Here's how the part is built. I have some questions about the finished solid (model axes, mm). A direction names the side the tool comes from. Round coordinates to 2 decimals unless told otherwise and drop trailing zeros. Write each loop counter-clockwise with the first axis right and the second up, starting at its lowest first coordinate (ties: lowest second). Pieces come first, ordered by that corner, then holes. Notation, with made-up numbers: (22, 22.25) - (50, 22.25) arc R26 ccw to (50, 59.25) - close; hole circle Ø4 at (26, 37.25). An arc over 180 degrees is marked (long way). Use one line per item in the form item = value. Start each with the question number.
1. I want a section at B-B, the plane z = 2. List the corners of the cut face in (x, y) for me, plus the area to 3 significant figures.
2. Will these pins go through, and if not, where does the flat tip stop? pin 1 (1 mm diameter, centred on y = 3, z = 6, fed in from -X); pin 2 (5 mm diameter, centred on x = -5.5, z = 6.5, fed in from +Y).
3. If I drill on line 1 along X through (y, z) = (0.4, -1.5); line 2 along Y through (x, z) = (6.25, 4); line 3 along Z through (x, y) = (-9.5, 3.7), over which ranges is the centre line in solid material (lowest first)?
4. Which directions (+Z, -Z, +X, -X, +Y, -Y) give clear straight access to the entire face, cutting with the end or side of a thin tool? Please do faces 1 (the flat face through (0, 2, -8.65)), 2 (the flat face through (-12, 1.6, 0)), 3 (the flat face through (0, 0, 0)), 4 (the flat face through (-11, 4, -3.8)), 5 (the flat face through (-11, 4, 3.8)).
5. I want a section at A-A, the plane x = -8.25. List the corners of the cut face in (y, z) for me, plus the area to 3 significant figures.
6. I want a section at C-C, the plane y = 3.95. List the corners of the cut face in (x, z) for me.
7. I want a section at D-D, the plane z = -7.25. List the corners of the cut face in (x, y) for me, plus the area to 3 significant figures.
```python
from build123d import *

# Parameters (mm, degrees)
SKETCH_1_W      = 23
SKETCH_1_H      = 17.3
EXTRUDE_1_DEPTH = 3.5
SKETCH_2_W      = 5.700101794
SKETCH_2_H      = 7.6
EXTRUDE_2_DEPTH = 0.7
SKETCH_3_W      = 1.500050897
SKETCH_3_H      = 7.6
EXTRUDE_3_DEPTH = 1.9


with BuildPart() as part:
    # Эскиз1 → Бобышка-Вытянуть1 (new body)
    with BuildSketch(Plane(origin=(0, 0, 0), x_dir=(1, 0, 0), z_dir=(0, 1, 0))):
        Rectangle(SKETCH_1_W, SKETCH_1_H)
    extrude(amount=EXTRUDE_1_DEPTH)

    # Эскиз2 → Бобышка-Вытянуть2 (add)
    with BuildSketch(Plane(origin=(0, 3.5, 0), x_dir=(1, 0, 0), z_dir=(0, 1, 0))):
        with Locations((-10.15, 0)):
            Rectangle(SKETCH_2_W, SKETCH_2_H)
    extrude(amount=EXTRUDE_2_DEPTH)

    # Эскиз3 → Бобышка-Вытянуть3 (add)
    with BuildSketch(Plane.XZ.offset(-3.5)):
        with Locations((-12.250025449, 0)):
            Rectangle(SKETCH_3_W, SKETCH_3_H)
    extrude(amount=EXTRUDE_3_DEPTH)


solid = part.part
```
Model answer:
q1.outline = (-13, 1.6) - (-11.5, 1.6) - (-11.5, 0) - (11.5, 0) - (11.5, 3.5) - (-7.3, 3.5) - (-7.3, 4.2) - (-13, 4.2) - close
q1.area = 87.3 mm2
q2.pin_1 = -11.5
q2.pin_2 = 3.5
q3.line_1 = -11.5 to 11.5
q3.line_2 = 0 to 3.5
q3.line_3 = -3.8 to 3.8
q4.face_1 = -Z, +X, -X, +Y, -Y
q4.face_2 = +Z, -Z, -X, -Y
q4.face_3 = +Z, -Z, +X, -X, -Y
q4.face_4 = -Z, -X, +Y
q4.face_5 = +Z, -X, +Y
q5.outline = (0, -8.65) - (3.5, -8.65) - (3.5, -3.8) - (4.2, -3.8) - (4.2, 3.8) - (3.5, 3.8) - (3.5, 8.65) - (0, 8.65) - close
q5.area = 65.9 mm2
q6.outline = (-13, -3.8) - (-7.3, -3.8) - (-7.3, 3.8) - (-13, 3.8) - close
q7.outline = (-11.5, 0) - (11.5, 0) - (11.5, 3.5) - (-11.5, 3.5) - close
q7.area = 80.5 mm2
